Design review of the part shown in the three views and the two pictorial views. Dimensions are in mm from the part's minimum x, y and z. A direction names the side the tool comes from. Coordinates: 2 decimals unless noted, no trailing zeros. Loops run counter-clockwise (first coordinate to the right, second up) from the corner with the lowest first, then second, coordinate; pieces in that order, holes last. Notation, with made-up numbers: M -17,-34.75 L 39,-34.75 A27 cw 39,-18.75 Z; hole C 76.5,-26.75 d7. An arc over 180 degrees is marked long. Use one line per item in the form item = value.
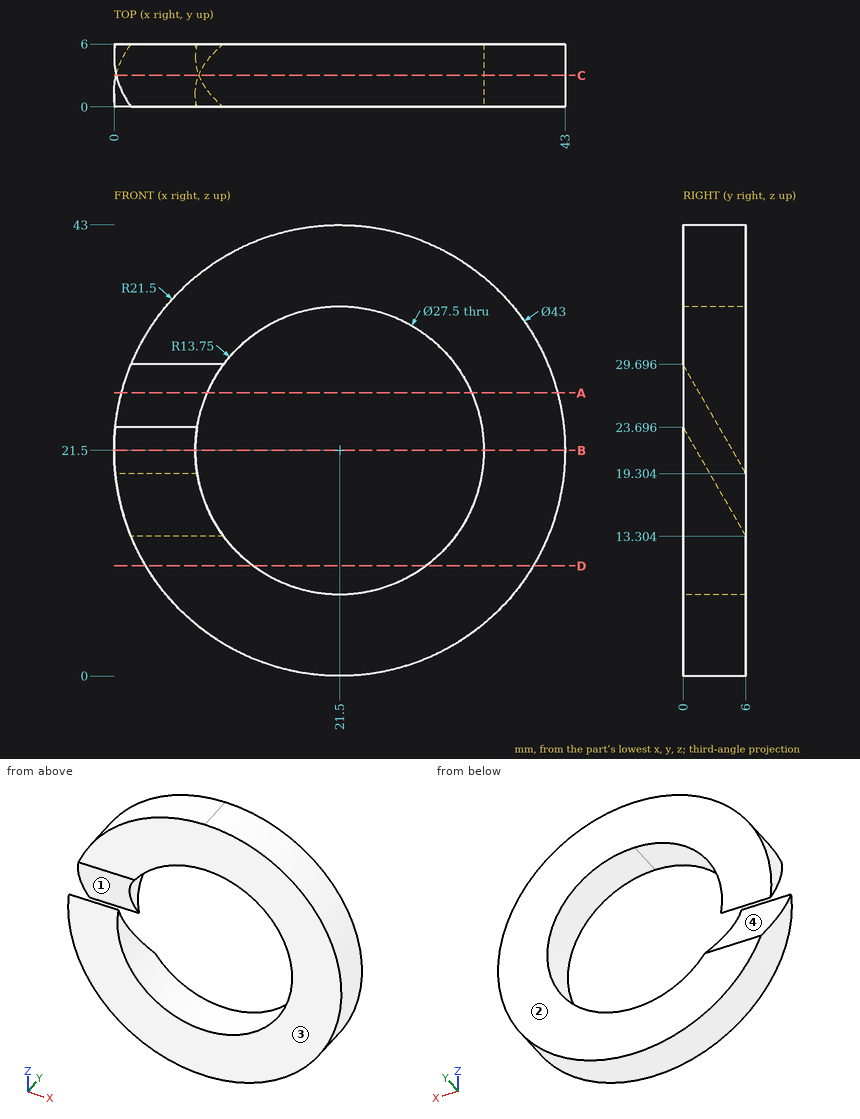
1. Add section B-B (z = 21.5). State the section outline as (x, y) points.
Response values:
outline = M 0,0 L 7.75,0 L 7.75,1.27 L 0,1.27 Z; M 0,4.73 L 7.75,4.73 L 7.75,6 L 0,6 Z; M 35.25,0 L 43,0 L 43,6 L 35.25,6 Z
2. The part is to be moulded in two halves that separate along Z. For the marked faces 3 and 4, say which applies: pulls with the +Z half, pulls with the -Z half, needs draft (parallel to the pull), parting line crosses it, or undercut.
Response values:
face_3 = needs draft
face_4 = undercut
3. Add section D-D (z = 10.5). State the section outline as (x, y) points.
Response values:
outline = M 3.03,0 L 13.25,0 L 13.25,6 L 3.03,6 Z; M 29.75,0 L 39.97,0 L 39.97,6 L 29.75,6 Z
4. Insertion check: P1, Ø2, axis at x = 24.5, y = 1.5, coming from the +Z side; P2, Ø1.5, axis at x = 16.5, y = 3.5, coming from the -Z side; P3, Ø1.5, axis at y = 0.5, z = 27.5, coming from the -X side. Each pin has a flat end and moves straight along its axis. Give the tip position at first contact, or say it passes through.
Response values:
P1 = 42.91
P2 = 0.42
P3 = 0.86
5. Add section A-A (z = 27). State the section outline as (x, y) points.
Response values:
outline = M 0.72,1.56 L 8.9,1.56 L 8.9,6 L 0.72,6 Z; M 34.1,0 L 42.28,0 L 42.28,6 L 34.1,6 Z
6. Wall thickness on line 1 along Z through (x, y) = (21.5, 1.75); line 2 along X through (y, z) = (1.5, 21.5); line 3 along X through (y, z) = (4.25, 22.5): over which ranges is each line inside the solid? List them lowest first. Write a range as from..to.
Response values:
line_1 = 0..7.75, 35.25..43
line_2 = 35.25..43
line_3 = 0.02..7.79, 35.21..42.98
7. Add section C-C (y = 3). State the section outline as (x, z) points.
Response values:
outline = M 0.21,18.5 A21.5 ccw long 0.21,24.5 L 8.08,24.5 A13.75 cw long 8.08,18.5 Z
8. Machinability: for the marked faces 1 and 2, which of the approach directions +Z, -Z, +X, -X, +Y, -Y give a long, thin tool a straight path to every point of the face, cutting with its end or side? Answer none if there is none.
Response values:
face_1 = -X
face_2 = +Z, -Z, +X, -X, +Y
